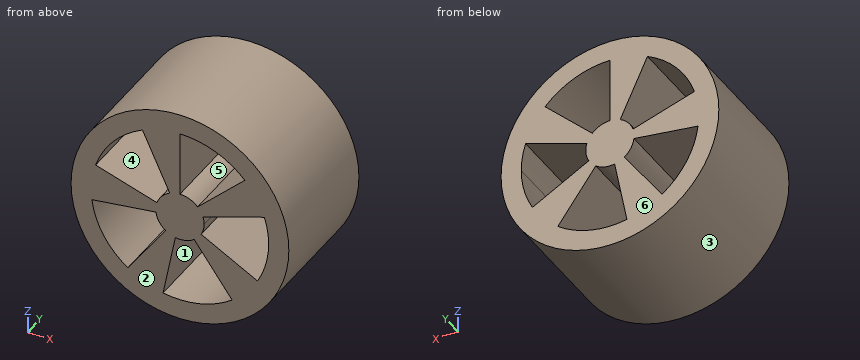
from build123d import *

# Parameters (mm, degrees)
F0_R     = 6.75
F1_DEPTH = 8
F3_DEPTH = 8


with BuildPart() as f1:
    # F0 (on Front) → F1 (new body)
    with BuildSketch(Plane.XZ):
        Circle(F0_R)
    extrude(amount=F1_DEPTH)

    # F2 (on Front) → F3 (cut)
    with BuildSketch(Plane.XZ):
        with BuildLine():
            ThreePointArc((1.426585, 0.463525), (1.481533, 0.234652), (1.5, 0))
            ThreePointArc((1.5, 0), (1.452221, -0.37557), (1.31193, -0.727214))
            Line((1.31193, -0.727214), (4.810408, -2.666453))
            ThreePointArc((4.810408, -2.666453), (5.324812, -1.37709), (5.5, 0))
            ThreePointArc((5.5, 0), (5.432286, 0.86039), (5.230811, 1.699593))
            Line((5.230811, 1.699593), (1.426585, 0.463525))
        make_face()
        with BuildLine():
            ThreePointArc((0, 1.5), (0.598124, 1.37559), (1.097031, 1.022998))
            Line((1.097031, 1.022998), (4.022445, 3.750991))
            ThreePointArc((4.022445, 3.750991), (2.19312, 5.04383), (0, 5.5))
            Line((0, 5.5), (0, 1.5))
        make_face()
        with BuildLine():
            ThreePointArc((-1.426585, 0.463525), (-1.123434, 0.99393), (-0.633927, 1.359462))
            Line((-0.633927, 1.359462), (-2.3244, 4.984693))
            ThreePointArc((-2.3244, 4.984693), (-4.119256, 3.64441), (-5.230811, 1.699593))
            Line((-5.230811, 1.699593), (-1.426585, 0.463525))
        make_face()
        with BuildLine():
            Line((3.232819, -4.449593), (0.881678, -1.213525))
            ThreePointArc((0.881678, -1.213525), (0.324659, -1.464444), (-0.286213, -1.472441))
            Line((-0.286213, -1.472441), (-1.049449, -5.39895))
            ThreePointArc((-1.049449, -5.39895), (1.190418, -5.369628), (3.232819, -4.449593))
        make_face()
        with BuildLine():
            Line((-3.232819, -4.449593), (-0.881678, -1.213525))
            ThreePointArc((-0.881678, -1.213525), (-1.292444, -0.761308), (-1.488819, -0.182804))
            Line((-1.488819, -0.182804), (-5.459004, -0.670281))
            ThreePointArc((-5.459004, -0.670281), (-4.73896, -2.791461), (-3.232819, -4.449593))
        make_face()
    extrude(amount=F3_DEPTH, mode=Mode.SUBTRACT)


solid = f1.part
Input: part model. Units: mm. Frame: model coordinates. Face numbers are marked on the shaded views. A direction names the side the tool comes from. Give positions to 0.01 mm unless a question says otherwise; leave off trailing zeros. Loops run counter-clockwise (first coordinate to the right, second up) from the corner with the lowest first, then second, coordinate; pieces in that order, holes last. Notation, with made-up numbers: (49, 62.5) -> (95, 62.5) arc R19 ccw to (95, 92.5) -> close; hole circle Ø7 at (25.5, -17). An arc over 180 degrees is marked (long way). Answer as a JSON object with one key per item and string values. Group by question number.
Item 1: Cut plane D-D, the plane x = -2.75. Return the cut outline in (y, z), and give its area (3 significant figures).
Item 2: Cut plane B-B, the plane z = -3.5. Return the cut outline in (x, y).
Item 3: Pin query (flat end, axial travel): P1, Ø1.5, axis at y = -6.5, z = -3, coming from the +X side; P2, Ø3, axis at x = -5, z = -1.5, coming from the -Y side; P3, Ø4, axis at x = -4, y = -1, coming from the -Z side. Return the tip coordinate at first contact, or that it passes through.
Item 4: Reachability of the marked faces 5 and 6 from +Z, -Z, +X, -X, +Y, -Y: full face, straight path, thin tool, end or side. Return the list, or none.
Item 5: Line query: probe 1 along Z at (x, y) = (-2.25, -0.5); probe 2 along Z at (x, y) = (1.25, -1.75); probe 3 along X at (y, z) = (-2.5, 3.5). Output: solid intervals per line, ascending.
Item 6: Cut plane C-C, the plane x = 5. Return the cut outline in (y, z), and give its area (3 significant figures).
Item 7: Pull-direction query (Z, two-part tool) for the marked faces 1, 2, 3 and 4; classes: released by +Z, released by -Z, zero draft, split by the parting line, or undercut.
Item 8: Cut plane A-A, the plane y = -2.5. Return the cut outline in (x, z).
Checks:
{
 "1": {"outline": "(-8, -6.16) -> (0, -6.16) -> (0, -3.79) -> (-8, -3.79) -> close; (-8, -0.34) -> (0, -0.34) -> (0, 0.89) -> (-8, 0.89) -> close; (-8, 4.76) -> (0, 4.76) -> (0, 6.16) -> (-8, 6.16) -> close", "area": "40.1 mm²"},
 "2": {"outline": "(-5.77, -8) -> (-4.24, -8) -> (-4.24, 0) -> (-5.77, 0) -> close; (-2.54, -8) -> (-0.68, -8) -> (-0.68, 0) -> (-2.54, 0) -> close; (2.54, -8) -> (5.77, -8) -> (5.77, 0) -> (2.54, 0) -> close"},
 "3": {"P1": "stops at x = 6.36", "P2": "stops at y = -8", "P3": "stops at z = -6.45"},
 "4": {"face 5": "+Y, -Y", "face 6": "+Z, -Z, +X, -X, +Y"},
 "5": {"probe 1": "z = -6.36 to -3.1, -0.28 to 0.73, 4.83 to 6.36", "probe 2": "z = -6.63 to -5.36, -1.72 to 1.17, 5.36 to 6.63", "probe 3": "x = -5.77 to -4.24, -1.63 to 0, 3.75 to 5.77"},
 "6": {"outline": "(-8, -4.53) -> (0, -4.53) -> (0, -2.29) -> (-8, -2.29) -> close; (-8, 1.62) -> (0, 1.62) -> (0, 4.53) -> (-8, 4.53) -> close", "area": "41.2 mm²"},
 "7": {"face 1": "undercut", "face 2": "zero draft", "face 3": "split by the parting line", "face 4": "undercut"},
 "8": {"outline": "circle Ø13.5 at (0, 0); hole (-5.46, -0.67) arc R5.5 ccw to (-3.23, -4.45) -> (-0.88, -1.21) arc R1.5 cw to (-1.49, -0.18) -> close; hole (-5.23, 1.7) -> (-1.43, 0.46) arc R1.5 cw to (-0.63, 1.36) -> (-2.32, 4.98) arc R5.5 ccw to start; hole (-1.05, -5.4) arc R5.5 ccw to (3.23, -4.45) -> (0.88, -1.21) arc R1.5 cw to (-0.29, -1.47) -> close; hole (0, 1.5) arc R1.5 cw to (1.1, 1.02) -> (4.02, 3.75) arc R5.5 ccw to (0, 5.5) -> close; hole (1.31, -0.73) -> (4.81, -2.67) arc R5.5 ccw to (5.5, 0) arc R5.5 ccw to (5.23, 1.7) -> (1.43, 0.46) arc R1.5 cw to (1.5, 0) arc R1.5 cw to start"}
}
